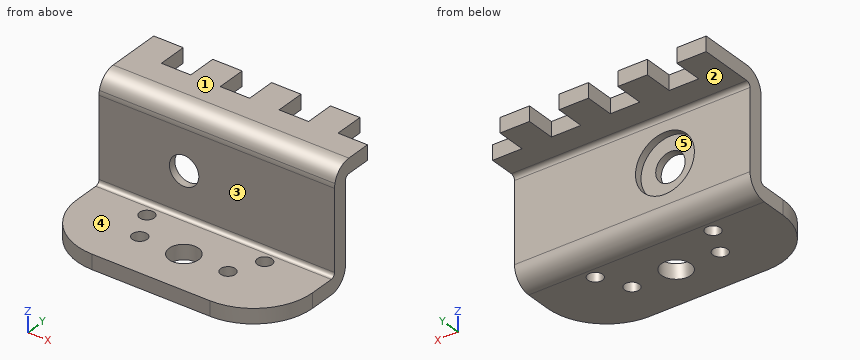
from build123d import *

# Parameters (mm, degrees)
SKETCH1_W           = 40
SKETCH1_H           = 50
SKETCH1_R           = 1.25
BASE_FLANGE1_DEPTH  = 2.5
SKETCH15_R          = 1
CUT_EXTRUDE3_DEPTH  = 10
JOG3_START          = -2.5
JOG3_OUTLINE_W      = 40
JOG3_OUTLINE_H      = 48.294687966
JOG3_OUTLINE_R      = 1
JOG3_OUTLINE_R_2    = 1.25
JOG3_DEPTH          = 2.5
JOG3_2_OUTLINE_W    = 40
JOG3_2_OUTLINE_H    = 1.705312034
JOG3_2_DEPTH        = 0.332528284
JOG3_START_2        = 14.2634
JOG3_3_OUTLINE_W    = 40
JOG3_3_OUTLINE_H    = 35
JOG3_3_OUTLINE_R    = 1
JOG3_3_OUTLINE_R_2  = 1.25
JOG3_3_DEPTH        = 3.2366
JOG3_4_OUTLINE_W    = 40
JOG3_4_OUTLINE_H    = 15.794687966
JOG3_4_OUTLINE_R    = 1.25
JOG3_4_DEPTH        = 3.2366
JOG3_5_OUTLINE_W    = 40
JOG3_5_OUTLINE_H    = 2.5
JOG3_5_DEPTH        = 15
JOG3_START_3        = 15
JOG3_6_OUTLINE_R    = 1.25
JOG3_6_OUTLINE_R_2  = 1
JOG3_6_DEPTH        = 2.5
JOG3_START_4        = -20
JOG3_7_DEPTH        = 40
JOG4_START          = -20
JOG4_DEPTH          = 40
JOG4_2_DEPTH        = 40
JOG4_START_2        = -3
JOG4_3_OUTLINE_R    = 1.25
JOG4_3_DEPTH        = 4
FILLET1_R           = 10
SKETCH18_R          = 2.5
BOSS_EXTRUDE1_DEPTH = 2.5
SKETCH19_R          = 1
SKETCH19_W          = 23.5
SKETCH19_H          = 12.5
CUT_EXTRUDE4_DEPTH  = 2.5
SKETCH20_R          = 2.5
SKETCH20_R_2        = 1.25
CUT_EXTRUDE6_DEPTH  = 10
SKETCH23_R          = 2.5
CUT_EXTRUDE7_DEPTH  = 44.945989578
SKETCH24_R          = 5
CUT_EXTRUDE8_DEPTH  = 1.25
SKETCH25_W          = 40
SKETCH25_H          = 18.401872862
CUT_EXTRUDE9_DEPTH  = 50.640775238


with BuildPart() as part:
    # Base-Flange1: sheet metal written as solids
    # Sketch1 → Base-Flange1 (new body)
    with BuildSketch(Plane.XY):
        Rectangle(SKETCH1_W, SKETCH1_H)
        with Locations((10, 12.5)):
            Circle(SKETCH1_R, mode=Mode.SUBTRACT)
        with Locations(Location((10, -12.5, 0), (0, 0, 180))):
            Circle(SKETCH1_R, mode=Mode.SUBTRACT)
        with Locations((-10, -12.5)):
            Circle(SKETCH1_R, mode=Mode.SUBTRACT)
        with Locations(Location((-10, 12.5, 0), (0, 0, 180))):
            Circle(SKETCH1_R, mode=Mode.SUBTRACT)
    extrude(amount=-BASE_FLANGE1_DEPTH)

    # Sketch15 → Cut-Extrude3 (cut)
    with BuildSketch(Plane.XY):
        with Locations((12, 0)):
            Circle(SKETCH15_R)
        with Locations(Location((-17, 0, 0), (0, 0, 180))):
            Circle(SKETCH15_R)
    extrude(amount=-CUT_EXTRUDE3_DEPTH, mode=Mode.SUBTRACT)

    # Jog3: read off the stored shape, not the designer's step
    # Jog3 outline → Jog3 (cut)
    with BuildSketch(Plane.XY.offset(JOG3_START)):
        with Locations((0, -0.852656017)):
            Rectangle(JOG3_OUTLINE_W, JOG3_OUTLINE_H)
        with Locations((-17, 0)):
            Circle(JOG3_OUTLINE_R, mode=Mode.SUBTRACT)
        with Locations((12, 0)):
            Circle(JOG3_OUTLINE_R, mode=Mode.SUBTRACT)
        with Locations((-10, 12.5)):
            Circle(JOG3_OUTLINE_R_2, mode=Mode.SUBTRACT)
        with Locations((10, 12.5)):
            Circle(JOG3_OUTLINE_R_2, mode=Mode.SUBTRACT)
        with Locations((10, -12.5)):
            Circle(JOG3_OUTLINE_R_2, mode=Mode.SUBTRACT)
        with Locations((-10, -12.5)):
            Circle(JOG3_OUTLINE_R_2, mode=Mode.SUBTRACT)
    extrude(amount=JOG3_DEPTH, mode=Mode.SUBTRACT)

    # Jog3 2 outline → Jog3 2 (cut)
    with BuildSketch(Plane.XY.offset(JOG3_START)):
        with Locations((0, 24.147343983)):
            Rectangle(JOG3_2_OUTLINE_W, JOG3_2_OUTLINE_H)
    extrude(amount=JOG3_2_DEPTH, mode=Mode.SUBTRACT)

    # Jog3 4 outline → Jog3 4 (add)
    with BuildSketch(Plane.XY.offset(JOG3_START)):
        with Locations((0, 32.897343983)):
            Rectangle(JOG3_4_OUTLINE_W, JOG3_4_OUTLINE_H)
        with Locations((10, 28.294687966)):
            Circle(JOG3_4_OUTLINE_R, mode=Mode.SUBTRACT)
        with Locations((-10, 28.294687966)):
            Circle(JOG3_4_OUTLINE_R, mode=Mode.SUBTRACT)
    extrude(amount=JOG3_4_DEPTH)



with BuildPart() as body_2:
    # Jog3 3 outline → Jog3 3 (new body)
    with BuildSketch(Plane.XY.offset(JOG3_START_2)):
        with Locations((0, 8.294687966)):
            Rectangle(JOG3_3_OUTLINE_W, JOG3_3_OUTLINE_H)
        with Locations((12, 15.794687966)):
            Circle(JOG3_3_OUTLINE_R, mode=Mode.SUBTRACT)
        with Locations((-17, 0)):
            Circle(JOG3_3_OUTLINE_R, mode=Mode.SUBTRACT)
        with Locations((-10, 3.294687966)):
            Circle(JOG3_3_OUTLINE_R_2, mode=Mode.SUBTRACT)
        with Locations((12, 0)):
            Circle(JOG3_3_OUTLINE_R, mode=Mode.SUBTRACT)
        with Locations((10, 3.294687966)):
            Circle(JOG3_3_OUTLINE_R_2, mode=Mode.SUBTRACT)
        with Locations((-17, 15.794687966)):
            Circle(JOG3_3_OUTLINE_R, mode=Mode.SUBTRACT)
        with Locations((-10, 12.5)):
            Circle(JOG3_3_OUTLINE_R_2, mode=Mode.SUBTRACT)
        with Locations((10, 12.5)):
            Circle(JOG3_3_OUTLINE_R_2, mode=Mode.SUBTRACT)
    extrude(amount=JOG3_3_DEPTH)


with BuildPart() as part_1:
    add(part.part)

    add(body_2.part)  # Jog3 5 merges body 2
    # Jog3 5 outline → Jog3 5 (add)
    with BuildSketch(Plane.XY):
        with Locations((0, 24.544687966)):
            Rectangle(JOG3_5_OUTLINE_W, JOG3_5_OUTLINE_H)
    extrude(amount=JOG3_5_DEPTH)

    # Jog3 6 outline → Jog3 6 (add)
    with BuildSketch(Plane.XY.offset(JOG3_START_3)):
        with Locations((10, 12.5)):
            Circle(JOG3_6_OUTLINE_R)
        with Locations((-10, 12.5)):
            Circle(JOG3_6_OUTLINE_R)
        with Locations((12, 0)):
            Circle(JOG3_6_OUTLINE_R_2)
        with Locations((-17, 0)):
            Circle(JOG3_6_OUTLINE_R_2)
    extrude(amount=JOG3_6_DEPTH)

    # Jog3 7 outline → Jog3 7 (cut)
    with BuildSketch(Plane.YZ.offset(JOG3_START_4)):
        with BuildLine():
            ThreePointArc((23.294687966, 14.2634), (23.078942821, 14.784254855), (22.558087966, 15))
            Line((22.558087966, 15), (-9.205312034, 15))
            Line((-9.205312034, 15), (-9.205312034, 14.2634))
            Line((-9.205312034, 14.2634), (23.294687966, 14.2634))
        make_face()
        with BuildLine():
            ThreePointArc((26.531287966, -2.5), (24.242666158, -1.552021808), (23.294687966, 0.7366))
            Line((23.294687966, 0.7366), (23.294687966, -2.167471716))
            Line((23.294687966, -2.167471716), (25, -2.167471716))
            Line((25, -2.167471716), (25, -2.5))
            Line((25, -2.5), (26.531287966, -2.5))
        make_face()
        with BuildLine():
            Line((26.531287966, 0), (40.794687966, 0))
            Line((40.794687966, 0), (40.794687966, 0.7366))
            Line((40.794687966, 0.7366), (25.794687966, 0.7366))
            ThreePointArc((25.794687966, 0.7366), (26.010433111, 0.215745145), (26.531287966, 0))
        make_face()
        with BuildLine():
            Line((25.794687966, 17.5), (22.558087966, 17.5))
            ThreePointArc((22.558087966, 17.5), (24.846709774, 16.552021808), (25.794687966, 14.2634))
            Line((25.794687966, 14.2634), (25.794687966, 17.5))
        make_face()
    extrude(amount=JOG3_7_DEPTH, mode=Mode.SUBTRACT)

    # Jog4: read off the stored shape, not the designer's step
    # Jog4 outline → Jog4 (cut)
    with BuildSketch(Plane.YZ.offset(JOG4_START)):
        with BuildLine():
            Line((-9.205312034, 15), (5.87962174, 15))
            ThreePointArc((5.87962174, 15), (7.019882984, 16.799110859), (9.031287966, 17.5))
            Line((9.031287966, 17.5), (-9.205312034, 17.5))
            Line((-9.205312034, 17.5), (-9.205312034, 15))
        make_face()
    extrude(amount=JOG4_DEPTH, mode=Mode.SUBTRACT)

    # Jog4 2 outline → Jog4 2 (add)
    with BuildSketch(Plane.YZ.offset(JOG4_START)):
        with BuildLine():
            Line((-9.205312034, 0), (-9.205312034, -2.5))
            Line((-9.205312034, -2.5), (5.058087966, -2.5))
            ThreePointArc((5.058087966, -2.5), (7.346709774, -1.552021808), (8.294687966, 0.7366))
            Line((8.294687966, 0.7366), (8.294687966, 14.2634))
            ThreePointArc((8.294687966, 14.2634), (8.510433111, 14.784254855), (9.031287966, 15))
            Line((9.031287966, 15), (5.87962174, 15))
            ThreePointArc((5.87962174, 15), (5.81599152, 14.634140241), (5.794687966, 14.2634))
            Line((5.794687966, 14.2634), (5.794687966, 0.7366))
            ThreePointArc((5.794687966, 0.7366), (5.578942821, 0.215745145), (5.058087966, 0))
            Line((5.058087966, 0), (-9.205312034, 0))
        make_face()
    extrude(amount=JOG4_2_DEPTH)

    # Jog4 3 outline → Jog4 3 (cut)
    with BuildSketch(Plane.XY.offset(JOG4_START_2)):
        with Locations((-10, 3.294687966)):
            Circle(JOG4_3_OUTLINE_R)
        with Locations((10, 3.294687966)):
            Circle(JOG4_3_OUTLINE_R)
    extrude(amount=JOG4_3_DEPTH, mode=Mode.SUBTRACT)

    # Fillet1
    fillet1_edges = [part_1.edges().sort_by_distance(p)[0] for p in [
        (20, -9.205312034, -1.25),
        (-20, -9.205312034, -1.25),
        (-20, 40.794687966, -1.25),
        (20, 40.794687966, -1.25),
    ]]
    fillet(fillet1_edges, radius=FILLET1_R)

    # Sketch18 → Boss-Extrude1 (add)
    with BuildSketch(Plane.XY.offset(17.5)):
        with Locations((12, 15.794687966)):
            Circle(SKETCH18_R)
        with Locations((-17, 15.794687966)):
            Circle(SKETCH18_R)
    extrude(amount=-BOSS_EXTRUDE1_DEPTH)

    # Sketch19 → Cut-Extrude4 (cut)
    with BuildSketch(Plane(origin=(0, 25.794687966, 0), x_dir=(1, 0, 0), z_dir=(0, 1, 0))):
        with Locations(Location((13.9, -7.5, 0), (0, 0, 270))):
            Circle(SKETCH19_R)
        with Locations(Location((-13.9, -7.5, 0), (0, 0, 90))):
            Circle(SKETCH19_R)
        with Locations((0, -7.5)):
            Rectangle(SKETCH19_W, SKETCH19_H)
    extrude(amount=-CUT_EXTRUDE4_DEPTH, mode=Mode.SUBTRACT)

    # Sketch20 → Cut-Extrude6 (cut)
    with BuildSketch(Plane.XY):
        with Locations((0, 33.294687966)):
            Circle(SKETCH20_R)
        with Locations(Location((0, -1.705312034, 0), (0, 0, 180))):
            Circle(SKETCH20_R)
        with Locations((7.5, -1.705312034)):
            Circle(SKETCH20_R_2)
        with Locations(Location((-7.5, -1.705312034, 0), (0, 0, 180))):
            Circle(SKETCH20_R_2)
        with Locations(Location((7.5, 33.294687966, 0), (0, 0, 180))):
            Circle(SKETCH20_R_2)
        with Locations((-7.5, 33.294687966)):
            Circle(SKETCH20_R_2)
    extrude(amount=-CUT_EXTRUDE6_DEPTH, mode=Mode.SUBTRACT)

    # Sketch23 → Cut-Extrude7 (cut, through all)
    with BuildSketch(Plane(origin=(0, 25.794687966, 0), x_dir=(1, 0, 0), z_dir=(0, 1, 0))):
        with Locations(Location((-5.55, -7.5, 0), (0, 0, 270))):
            Circle(SKETCH23_R)
    extrude(amount=-CUT_EXTRUDE7_DEPTH, mode=Mode.SUBTRACT)

    # Sketch24 → Cut-Extrude8 (cut)
    with BuildSketch(Plane(origin=(0, 8.294687966, 0), x_dir=(1, 0, 0), z_dir=(0, 1, 0))):
        with Locations(Location((-5.55, -7.5, 0), (0, 0, 270))):
            Circle(SKETCH24_R)
    extrude(amount=-CUT_EXTRUDE8_DEPTH, mode=Mode.SUBTRACT)

    # Sketch25 → Cut-Extrude9 (cut, through all)
    with BuildSketch(Plane.XY.offset(17.5)):
        Polygon((-20, 22.558087966), (-20, 18.294687966), (-15, 18.294687966), (-15, 13.294687966), (-10, 13.294687966), (-10, 15.794687966), (-10, 18.294687966), (-5, 18.294687966), (-5, 13.294687966), (0, 13.294687966), (0, 15.794687966), (0, 18.294687966), (5, 18.294687966), (5, 13.294687966), (10, 13.294687966), (10, 15.794687966), (10, 18.294687966), (15, 18.294687966), (15, 13.294687966), (20, 13.294687966), (20, 15.794687966), (20, 22.558087966), align=None)
        with Locations((0, 31.759024397)):
            Rectangle(SKETCH25_W, SKETCH25_H)
    extrude(amount=-CUT_EXTRUDE9_DEPTH, mode=Mode.SUBTRACT)


solid = part_1.part
The listing builds one solid part. Answer for the finished solid, in the listing's coordinates (mm). Face numbers are marked on the shaded views. A direction names the side the tool comes from. Coordinates: 2 decimals unless noted, no trailing zeros. Loops run counter-clockwise (first coordinate to the right, second up) from the corner with the lowest first, then second, coordinate; pieces in that order, holes last. Notation, with made-up numbers: M -26,64.25 L -20,64.25 A15 cw -20,79.25 Z; hole C 41,7 d5. An arc over 180 degrees is marked long. Answer in a Markdown table with one row per item.
1) Given pin 1 (3 mm diameter, centred on x = -13, z = 8.5, fed in from -Y); pin 2 (4 mm diameter, centred on x = -10, y = 3.29, fed in from -Z); pin 3 (6 mm diameter, centred on x = 9, z = 2, fed in from +Y); pin 4 (7 mm diameter, centred on x = -6.5, y = -5.5, fed in from +Z), each flat-ended and moving along its own axis, determine where each tip first touches the part or whether it passes through.
Answers below:
| item | result |
|---|---|
| pin 1 | y = 5.79 |
| pin 2 | z = -2.5 |
| pin 3 | y = 8.29 |
| pin 4 | z = 0 |
2) Find section C-C (x = -5.55). Determine the outline of the cut face in (y, z).
Answers below:
| item | result |
|---|---|
| outline | M -9.21,-2.5 L 5.06,-2.5 A3.24 ccw 8.29,0.74 L 8.29,2.5 L 7.04,2.5 L 7.04,5 L 5.79,5 L 5.79,0.74 A0.74 cw 5.06,0 L -9.21,0 Z; M 5.79,10 L 7.04,10 L 7.04,12.5 L 8.29,12.5 L 8.29,14.26 A0.74 cw 9.03,15 L 18.29,15 L 18.29,17.5 L 9.03,17.5 A3.24 ccw 5.79,14.26 Z |
3) Find section A-A (y = 15). Determine the outline of the cut face in (x, z).
Answers below:
| item | result |
|---|---|
| outline | M -20,15 L -15,15 L -15,17.5 L -20,17.5 Z; M -10,15 L -5,15 L -5,17.5 L -10,17.5 Z; M 0,15 L 5,15 L 5,17.5 L 0,17.5 Z; M 10,15 L 15,15 L 15,17.5 L 10,17.5 Z |
4) Find section D-D (x = 4). Determine the outline of the cut face in (y, z).
Answers below:
| item | result |
|---|---|
| outline | M -9.21,-2.5 L 5.06,-2.5 A3.24 ccw 8.29,0.74 L 8.29,14.26 A0.74 cw 9.03,15 L 18.29,15 L 18.29,17.5 L 9.03,17.5 A3.24 ccw 5.79,14.26 L 5.79,0.74 A0.74 cw 5.06,0 L -9.21,0 Z |
5) Determine the mould class of the marked faces 4 and 5 for opening direction X: released by +X, released by -X, zero draft, split by the parting line, or undercut.
Answers below:
| item | result |
|---|---|
| face 4 | zero draft |
| face 5 | undercut |
6) Find section B-B (z = 7.5). Determine the outline of the cut face in (x, y), then the cut area to 4 significant figures.
Answers below:
| item | result |
|---|---|
| outline | M -20,5.79 L -8.05,5.79 L -8.05,7.04 L -10.55,7.04 L -10.55,8.29 L -20,8.29 Z; M -3.05,5.79 L 20,5.79 L 20,8.29 L -0.55,8.29 L -0.55,7.04 L -3.05,7.04 Z |
| area | 81.25 mm^2 |
7) Find the intervals of material crossed by probe 1 along X at (y, z) = (6.3, 7.5); probe 2 along Z at (x, y) = (16, 9); probe 3 along Z at (x, y) = (-10.5, -2.25), in increasing order.
Answers below:
| item | result |
|---|---|
| probe 1 | -20 to -8.05, -3.05 to 20 |
| probe 2 | 15 to 17.5 |
| probe 3 | -2.5 to 0 |
8) Which of the six approach directions +Z, -Z, +X, -X, +Y, -Y give full straight-line access (tool end or side, diameter ignored) to the marked faces 1, 2 and 3?
Answers below:
| item | result |
|---|---|
| face 1 | +Z, +X, -X, +Y, -Y |
| face 2 | -Z, +X, -X, +Y |
| face 3 | +Z, +X, -X, -Y |
